Autodesk Inventor part; units mm, degrees
ref_plane "YZ Plane" through (0, 0, 0) normal (1, 0, 0) x (0, 1, 0)
ref_plane "XZ Plane" through (0, 0, 0) normal (0, 1, 0) x (-1, 0, 0)
ref_plane "XY Plane" through (0, 0, 0) normal (0, 0, 1) x (1, 0, 0)
sketch "Sketch1" plane through (0, 0, 0) normal (0, 0, 1) x (1, 0, 0)
  line L0 (-38.5, 36) -> (38.5, 36)
  line L1 (38.5, 36) -> (38.5, -36)
  line L2 (38.5, -36) -> (-38.5, -36)
  line L3 (-38.5, -36) -> (-38.5, 36)
  line L4 (-38.5, 36) -> (38.5, -36) construction
  line L5 (38.5, 36) -> (-38.5, -36) construction
  circle A0 centre (0, 31.1) radius 1.6
  point P0 (0, 0)
  dimension "d0" = 72
  dimension "d1" = 77
  dimension "d24" = 3.2
  dimension "d25" = 4.9
sketch "Sketch2" plane through (0, 0, 1) normal (0, 0, 1) x (1, 0, 0)
  line L0 (-38.5, 36) -> (38.5, 36)
  line L1 (-48.5, 26) -> (-38.5, 26)
  line L2 (-38.5, 26) -> (-38.5, 36)
  line L3 (-38.5, 36) -> (-48.5, 36)
  line L4 (-48.5, 36) -> (-48.5, 26)
  line L5 (-48.5, 26) -> (-38.5, 36) construction
  line L6 (-38.5, 26) -> (-48.5, 36) construction
  line L7 (0, 0) -> (0, 7.0571)
  line L8 (0, 0) -> (6.6312, 0)
  line L9 (-38.5, -36) -> (-38.5, 36)
  line L10 (48.5, 26) -> (38.5, 26)
  line L11 (38.5, 26) -> (38.5, 36)
  line L12 (38.5, 36) -> (48.5, 36)
  line L13 (48.5, 36) -> (48.5, 26)
  line L14 (48.5, 26) -> (38.5, 36) construction
  line L15 (38.5, 26) -> (48.5, 36) construction
  circle A0 centre (-44.5, 31) radius 1.6
  circle A1 centre (44.5, 31) radius 1.6
  line L16 (38.5, -36) -> (-38.5, -36)
  line L17 (-5, -46) -> (5, -46)
  line L18 (5, -46) -> (5, -36)
  line L19 (5, -36) -> (-5, -36)
  line L20 (-5, -36) -> (-5, -46)
  line L21 (-5, -46) -> (5, -36) construction
  line L22 (5, -46) -> (-5, -36) construction
  circle A2 centre (0, -42) radius 1.6
  line L23 (-48.5, -26) -> (-38.5, -26)
  line L24 (-38.5, -26) -> (-38.5, -36)
  line L25 (-38.5, -36) -> (-48.5, -36)
  line L26 (-48.5, -36) -> (-48.5, -26)
  line L27 (-48.5, -26) -> (-38.5, -36) construction
  line L28 (-38.5, -26) -> (-48.5, -36) construction
  line L29 (38.5, -26) -> (38.5, -36)
  line L30 (38.5, -36) -> (48.5, -36)
  line L31 (48.5, -36) -> (48.5, -26)
  line L32 (48.5, -26) -> (38.5, -36) construction
  line L33 (38.5, -26) -> (48.5, -36) construction
  line L34 (48.5, -26) -> (38.5, -26)
  circle A3 centre (-44.5, -31) radius 1.6
  circle A4 centre (44.5, -31) radius 1.6
  point P0 (-43.5, 31)
  point P1 (43.5, 31)
  point P2 (0, -41)
  point P3 (-38.5, -36)
  point P4 (-43.5, -31)
  point P5 (43.5, -31)
  dimension "d5" = 10
  dimension "d6" = 10
  dimension "d10" = 3.2
  dimension "d12" = 4
  dimension "d18" = 3.2
  dimension "d19" = 10
  dimension "d20" = 10
  dimension "d21" = 4
  dimension "d22" = 5
extrude "Plate1" add sketch "Sketch1" along normal blind 1
sheet face with bend "Face2" sketch "Sketch2" thickness 1 toward (0, 0, -1) bend radius 1
bend "Bend1"
equation "\"d2\" = 厚度"
equation "\"d13\" = 折彎半徑"
equation "\"d14\" = 折彎離隙寬度"
equation "\"d16\" = 最小剩餘"
equation "\"d15\" = 折彎離隙深度"
equation "\"d17\" = 轉移半徑"
equation "\"折彎半徑\" = 厚度"
equation "\"折彎離隙寬度\" = 厚度"
equation "\"折彎離隙深度\" = 0.5 * 厚度"
equation "\"轉角離隙大小\" = 4 * 厚度"
equation "\"最小剩餘\" = 2 * 厚度"
equation "\"轉移半徑\" = 折彎半徑"
equation "\"Jacobi半徑大小\" = 折彎半徑"
equation "\"間隙大小\" = 厚度"
properties part number "battery_box_24V_base" material "Aluminum"
Verification items for the finished model (mm, model axes). Round coordinates to 2 decimals unless told otherwise and drop trailing zeros. Loops run counter-clockwise (first coordinate to the right, second up) from the corner with the lowest first, then second, coordinate; pieces in that order, holes last. Notation, with made-up numbers: (24, 20.5) - (45, 20.5) arc R15 ccw to (45, 39.5) - close; hole circle Ø10 at (23, -25). An arc over 180 degrees is marked (long way). Write item = value, one per line.
Q1. Mould release check, pull along X, two halves, no side actions. Record for faces 1 (the flat face through (-1, -4, 0)), 2 (the cylindrical face through (45.24, -32.42, 0.51)): +X half, -X half, draft (parallel to the pull), parting line (faces both ways), or undercut.
Here are the results:
face_1 = draft
face_2 = undercut
Q2. Material ranges on L1, parallel to Y at x = -44.5, z = 0.45; L2, parallel to Y at x = -1, z = 0.35; L3, parallel to Y at x = -39, z = 0.6, recorded low to high.
Here are the results:
L1 = -36 to -32.6, -29.4 to -26, 26 to 29.4, 32.6 to 36
L2 = -46 to -43.25, -40.75 to 29.85, 32.35 to 36
L3 = -36 to -26, 26 to 36
Q3. Sectioned sample at D-D on x = 44.5. Record the boundary of the cut face in (y, z).
Here are the results:
outline = (-36, 0) - (-32.6, 0) - (-32.6, 1) - (-36, 1) - close; (-29.4, 0) - (-26, 0) - (-26, 1) - (-29.4, 1) - close; (26, 0) - (29.4, 0) - (29.4, 1) - (26, 1) - close; (32.6, 0) - (36, 0) - (36, 1) - (32.6, 1) - close
Q4. Sectioned sample at A-A on z = 0.2. Record the boundary of the cut face in (x, y).
Here are the results:
outline = (-48.5, -36) - (-5, -36) - (-5, -46) - (5, -46) - (5, -36) - (48.5, -36) - (48.5, -26) - (38.5, -26) - (38.5, 26) - (48.5, 26) - (48.5, 36) - (-48.5, 36) - (-48.5, 26) - (-38.5, 26) - (-38.5, -26) - (-48.5, -26) - close; hole circle Ø3.2 at (-44.5, -31); hole circle Ø3.2 at (-44.5, 31); hole circle Ø3.2 at (0, -42); hole circle Ø3.2 at (0, 31.1); hole circle Ø3.2 at (44.5, -31); hole circle Ø3.2 at (44.5, 31)
Q5. Sectioned sample at C-C on x = 0. Record the boundary of the cut face in (y, z).
Here are the results:
outline = (-46, 0) - (-43.6, 0) - (-43.6, 1) - (-46, 1) - close; (-40.4, 0) - (29.5, 0) - (29.5, 1) - (-40.4, 1) - close; (32.7, 0) - (36, 0) - (36, 1) - (32.7, 1) - close
Q6. Depth check by flat-ended pin: pin 1 (0.5 mm diameter, centred on y = 3.5, z = 0.5, fed in from -X). Enter the tip coordinate at first touch or a pass-through.
Here are the results:
pin_1 = -38.5
Q7. Sectioned sample at B-B on y = -31. Record the boundary of the cut face in (x, z).
Here are the results:
outline = (-48.5, 0) - (-46.1, 0) - (-46.1, 1) - (-48.5, 1) - close; (-42.9, 0) - (42.9, 0) - (42.9, 1) - (-42.9, 1) - close; (46.1, 0) - (48.5, 0) - (48.5, 1) - (46.1, 1) - close
